Geometry: final body of the model. Coordinates: model frame, mm. Face numbers are marked on the shaded views. A direction names the side the tool comes from. Give positions to 0.01 mm unless a question says otherwise; leave off trailing zeros. Loops run counter-clockwise (first coordinate to the right, second up) from the corner with the lowest first, then second, coordinate; pieces in that order, holes last.
1. Draft query along Z for the marked faces 3, 4, 5 and 6. Return one class per face: +Z half, -Z half, draft (parallel to the pull), parting line (faces both ways), or undercut.
2. Material intervals for line 1 along X through (y, z) = (12.75, -5.5); line 2 along Z through (x, y) = (13, 12.75); line 3 along X through (y, z) = (7.25, 24), sorted ascending.
3. First-contact query: P1, Ø9, axis at x = 12.5, y = 7, coming from the +Z side; P2, Ø2, axis at x = -9, z = 9.5, coming from the +Y side; P3, Ø5.5, axis at y = 13, z = 2.5, coming from the -X side. Flat tips, straight axial feed; report the tip coordinate or a pass-through.
4. Section C-C, the plane z = -14. Output: boundary loops of the cut face in (x, y), then the cut area to 3 significant figures.
5. Access query for the marked faces 1 and 2. Directions: +Z, -Z, +X, -X, +Y, -Y. A direction counts if a zero-diameter tool reaches every point of the face in a straight line with its end or side. Return the directions, or none.
6. Section A-A, the plane y = 13.25. Output: boundary loops of the cut face in (x, z), then the cut area to 3 significant figures.
7. Section B-B, the plane x = 14. Output: boundary loops of the cut face in (y, z), then the cut area to 3 significant figures.
from build123d import *

# Parameters (mm, degrees)
SKETCH1_W                       = 116
SKETCH1_H                       = 60
SKETCH1_W_2                     = 110
SKETCH1_H_2                     = 54
BOSS_EXTRUDE1_DEPTH             = 10
SKETCH2_W                       = 116
SKETCH2_H                       = 60
BOSS_EXTRUDE2_DEPTH             = 3
CUT_EXTRUDE1_DEPTH              = 12.5
BOSS_EXTRUDE4_REACH             = 68.061
BOSS_EXTRUDE4_DIRECTION_2_REACH = 68.061
BOSS_EXTRUDE5_DEPTH             = 55
CUT_EXTRUDE2_DEPTH              = 4
SKETCH7_W                       = 113
SKETCH7_H                       = 57
SKETCH7_W_2                     = 110
SKETCH7_H_2                     = 54
BOSS_EXTRUDE6_DEPTH             = 5


with BuildPart() as part:
    # Sketch1 → Boss-Extrude1 (new body)
    with BuildSketch(Plane(origin=(0, 0, 0), x_dir=(1, 0, 0), z_dir=(0, 1, 0))):
        Rectangle(SKETCH1_W, SKETCH1_H)
        Rectangle(SKETCH1_W_2, SKETCH1_H_2, mode=Mode.SUBTRACT)
    extrude(amount=BOSS_EXTRUDE1_DEPTH)

    # Sketch2 → Boss-Extrude2 (add)
    with BuildSketch(Plane.XZ):
        Rectangle(SKETCH2_W, SKETCH2_H)
    extrude(amount=BOSS_EXTRUDE2_DEPTH)

    # Sketch3 → Cut-Extrude1 (cut, symmetric)
    with BuildSketch(Plane(origin=(0, 0, 0), x_dir=(0, 0, -1), z_dir=(1, 0, 0))):
        Polygon((-28.5, 10), (-31, 10), (-31, 4), (-28.5, 6.5), (-28.5, 7.5), (-30, 7.5), (-30, 8.5), align=None)
    cut_extrude1 = extrude(amount=CUT_EXTRUDE1_DEPTH, both=True, mode=Mode.SUBTRACT)

    # Mirror1: Cut-Extrude1 across plane
    add(cut_extrude1.mirror(Plane.XY), mode=Mode.SUBTRACT)

    # Boss-Extrude4: up to this face of the body (flat: up to its plane)
    boss_extrude4_end = Plane(part.part.faces().sort_by_distance((58, 3.5, 0))[0])
    # Sketch4 → Boss-Extrude4 (add, up to the picked face)
    with BuildSketch(Plane(origin=(0, 0, 0), x_dir=(0, 0, -1), z_dir=(1, 0, 0)), mode=Mode.PRIVATE) as boss_extrude4_sk1:
        with BuildLine():
            Line((30, 2), (30, -3))
            ThreePointArc((30, -3), (32.5, -0.5), (30, 2))
        make_face()
    boss_extrude4_tool1 = split(extrude(boss_extrude4_sk1.sketch, amount=BOSS_EXTRUDE4_REACH, mode=Mode.PRIVATE), bisect_by=boss_extrude4_end, keep=Keep.BOTH, mode=Mode.PRIVATE)
    boss_extrude4 = boss_extrude4_tool1.solids().sort_by(Axis((0, -0.5, -31.061033), (1, 0, 0)))[0]
    add(boss_extrude4)

    # Boss-Extrude4 direction 2: up to this face of the body (flat: up to its plane)
    boss_extrude4_direction_2_end = Plane(part.part.faces().sort_by_distance((-58, 3.5, 0))[0])
    # Sketch4 → Boss-Extrude4 direction 2 (add, up to the picked face)
    with BuildSketch(Plane(origin=(0, 0, 0), x_dir=(0, 0, -1), z_dir=(1, 0, 0)), mode=Mode.PRIVATE) as boss_extrude4_direction_2_sk1:
        with BuildLine():
            Line((30, 2), (30, -3))
            ThreePointArc((30, -3), (32.5, -0.5), (30, 2))
        make_face()
    boss_extrude4_direction_2_tool1 = split(extrude(boss_extrude4_direction_2_sk1.sketch, amount=-BOSS_EXTRUDE4_DIRECTION_2_REACH, mode=Mode.PRIVATE), bisect_by=boss_extrude4_direction_2_end, keep=Keep.BOTH, mode=Mode.PRIVATE)
    boss_extrude4_direction_2 = boss_extrude4_direction_2_tool1.solids().sort_by(Axis((0, -0.5, -31.061033), (-1, 0, 0)))[0]
    add(boss_extrude4_direction_2)

    # Mirror3: Boss-Extrude4, Boss-Extrude4 direction 2 across plane
    add(boss_extrude4.mirror(Plane.XY))
    add(boss_extrude4_direction_2.mirror(Plane.XY))


with BuildPart() as body_2:
    # Sketch5 → Boss-Extrude5 (new, symmetric)
    with BuildSketch(Plane(origin=(0, 0, 0), x_dir=(0, 0, -1), z_dir=(1, 0, 0))):
        with BuildLine():
            Line((26.787564435, -2.3), (26.383419246, -3))
            Line((26.383419246, -3), (28, -3))
            ThreePointArc((28, -3), (29.996934481, -0.214678652), (32.5, 2.126352177))
            Line((32.5, 2.126352177), (32.5, 3.852866185))
            ThreePointArc((32.5, 3.852866185), (29.29668765, 1.098682153), (26.787564435, -2.3))
        make_face()
    extrude(amount=BOSS_EXTRUDE5_DEPTH, both=True)

    # Sketch6 → Cut-Extrude2 (cut, symmetric)
    with BuildSketch(Plane(origin=(0, 0, 0), x_dir=(0, 0, -1), z_dir=(1, 0, 0))):
        with BuildLine():
            Line((26.383419246, -3), (28, -3))
            ThreePointArc((28, -3), (29.996934481, -0.214678652), (32.5, 2.126352177))
            Line((32.5, 2.126352177), (32.5, 3.852866185))
            ThreePointArc((32.5, 3.852866185), (29.29668765, 1.098682153), (26.787564435, -2.3))
            Line((26.787564435, -2.3), (26.383419246, -3))
        make_face()
    extrude(amount=CUT_EXTRUDE2_DEPTH, both=True, mode=Mode.SUBTRACT)


with BuildPart() as cut_extrude2_piece_1:
    # of the separate pieces the step leaves, piece 1, a body of its own (cut_extrude2_pieces)
    add(body_2.part.solids().sort_by_distance((-4, -2.3, -26.787564435))[0])


with BuildPart() as cut_extrude2_piece_2:
    # of the separate pieces the step leaves, piece 2, a body of its own (cut_extrude2_pieces)
    add(body_2.part.solids().sort_by_distance((55, -2.3, -26.787564435))[0])


with BuildPart() as body_4:
    # Mirror2: mirrored copy
    add(cut_extrude2_piece_1.part.mirror(Plane.XY))


with BuildPart() as body_5:
    # Mirror2 2: mirrored copy
    add(cut_extrude2_piece_2.part.mirror(Plane.XY))


with BuildPart() as part_1:
    add(part.part)

    # Combine2: cut Cut-Extrude2 piece 1, Cut-Extrude2 piece 2, body 5, body 4
    add(cut_extrude2_piece_1.part, mode=Mode.SUBTRACT)
    add(cut_extrude2_piece_2.part, mode=Mode.SUBTRACT)
    add(body_5.part, mode=Mode.SUBTRACT)
    add(body_4.part, mode=Mode.SUBTRACT)

    # Sketch7 → Boss-Extrude6 (add)
    with BuildSketch(Plane(origin=(0, 10, 0), x_dir=(1, 0, 0), z_dir=(0, 1, 0))):
        Rectangle(SKETCH7_W, SKETCH7_H)
        Rectangle(SKETCH7_W_2, SKETCH7_H_2, mode=Mode.SUBTRACT)
    extrude(amount=BOSS_EXTRUDE6_DEPTH)


solid = part_1.part
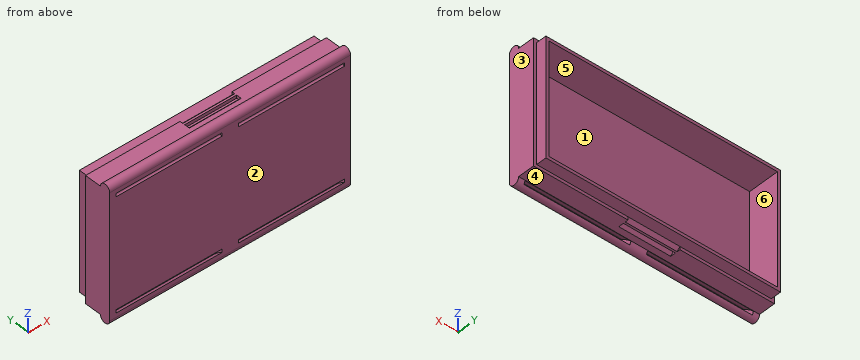
Answers below:
1. face 3: draft
1. face 4: -Z half
1. face 5: undercut
1. face 6: undercut
2. line 1: x = -56.5 to -55, 55 to 56.5
2. line 2: z = -28.5 to -27, 27 to 28.5
2. line 3: x = -58 to -55, 55 to 58
3. P1: stops at z = 30
3. P2: stops at y = 0
3. P3: stops at x = -56.5
4. outline: (-58, -3) - (58, -3) - (58, 10) - (56.5, 10) - (56.5, 15) - (55, 15) - (55, 0) - (-55, 0) - (-55, 15) - (-56.5, 15) - (-56.5, 10) - (-58, 10) - close
4. area: 423 mm2
5. face 1: +Y
5. face 2: +Z, -Z, +X, -X, -Y
6. outline: (-56.5, -28.5) - (56.5, -28.5) - (56.5, 28.5) - (-56.5, 28.5) - close; hole (-55, -27) - (55, -27) - (55, 27) - (-55, 27) - close
6. area: 501 mm2
7. outline: (-3, -30) arc R2.5 ccw to (1.4, -31.62) arc R17.44 ccw to (-3, -28) - close; (-3, -26.38) - (-2.3, -26.79) arc R18.84 cw to (1.99, -30.18) arc R2.5 ccw to (2, -30) - (10, -30) - (10, -28.5) - (15, -28.5) - (15, -27) - (0, -27) - (0, 27) - (15, 27) - (15, 28.5) - (10, 28.5) - (10, 30) - (2, 30) arc R2.5 ccw to (1.99, 30.18) arc R18.84 cw to (-2.3, 26.79) - (-3, 26.38) - close; (-3, 28) arc R17.44 ccw to (1.4, 31.62) arc R2.5 ccw to (-3, 30) - close
7. area: 258 mm2
